Design review of the part built by this model. Coordinates are the model's own, in mm. A direction names the side the tool comes from. Round coordinates to 2 decimals unless told otherwise and drop trailing zeros. Loops run counter-clockwise (first coordinate to the right, second up) from the corner with the lowest first, then second, coordinate; pieces in that order, holes last. Notation, with made-up numbers: M 32.25,23.25 L 38.25,23.25 A29 ccw 38.25,51.25 Z; hole C 72,69.25 d1. An arc over 180 degrees is marked long. One line per item, written item: value. Start each with the question number.
Item 1: We need section C-C (x = 19). Write out the cut boundary in (y, z).
Item 2: Clearance check with a flat-ended pin moving along its axis: pin 1 (1.5 mm diameter, centred on x = -19.5, y = 23.5, fed in from +Z). State where the tip first meets the part, or that it passes through.
Item 3: For faces 1 (the flat face through (-18, 36.594, 31)), 2 (the flat face through (-68.472, -2, 28)), list the 3-axis set-ups (+Z, -Z, +X, -X, +Y, -Y) from which the entire face can be reached by the end or side of a thin tool; tool diameter is ignored.
Item 4: For line 1 along Y through (x, z) = (2.5, 17.5); line 2 along X through (y, z) = (-20, 40); line 3 along Z through (x, y) = (-32, -36), list the stretches that pass through material, from the lowest coordinate up.
Item 5: We need section A-A (z = 9.5). Write out the cut boundary in (x, y).
Item 6: Mouldability with a two-part tool opening along Y and no side actions: class faces 3 (the flat face through (-18, -46.271, 28)), 4 (the flat face through (-16, -41.152, 31)), 5 (the flat face through (-17, 41.641, 28)), 6 (the flat face through (-62.202, -3, 31)) as released by +Y, released by -Y, zero draft, split by the parting line, or undercut.
Item 7: We need section B-B (y = -36). Write out the cut boundary in (x, z), then the cut area to 3 significant figures.
from build123d import *

# Parameters (mm, degrees)
F0_W     = 90.4587376863
F0_H     = 77.7452811599
F1_DEPTH = 6.35
F0_W_2   = 5.1199775189
F2_DEPTH = 55.88


with BuildPart() as f1:
    # F0 (on Top) → F1 (new body)
    with BuildSketch(Plane.XY):
        with Locations((-16.9725483283, -2.2788867354)):
            Rectangle(F0_W, F0_H)
    extrude(amount=F1_DEPTH)

    # F0 (on Top) → F2 (join)
    with BuildSketch(Plane.XY):
        Polygon((-62.2019171715, 41.6413508356), (-62.2019171715, 36.5937538445), (28.2568205148, 36.5937538445), (33.3767980337, 36.5937538445), (33.3767980337, 41.6413508356), align=None)
        Polygon((-62.2019171715, -41.1515273154), (-62.2019171715, 36.5937538445), (-62.2019171715, 41.6413508356), (-68.4723928571, 41.6413508356), (-68.4723928571, -46.2711900473), (-62.2019171715, -46.2711900473), align=None)
        with Locations((30.8168092743, -2.2788867354)):
            Rectangle(F0_W_2, F0_H)
        Polygon((28.2568205148, -41.1515273154), (-62.2019171715, -41.1515273154), (-62.2019171715, -46.2711900473), (33.3767980337, -46.2711900473), (33.3767980337, -41.1515273154), align=None)
    extrude(amount=F2_DEPTH)


solid = f1.part
A:
1. outline: M -46.27,0 L 41.64,0 L 41.64,55.88 L 36.59,55.88 L 36.59,6.35 L -41.15,6.35 L -41.15,55.88 L -46.27,55.88 Z
2. pin 1: z = 6.35
3. face 1: +Z
3. face 2: +Z, -Z, -X, +Y, -Y
4. line 1: -46.27 to -41.15, 36.59 to 41.64
4. line 2: -68.47 to -62.2, 28.26 to 33.38
4. line 3: 0 to 6.35
5. outline: M -68.47,-46.27 L 33.38,-46.27 L 33.38,41.64 L -68.47,41.64 Z; hole M -62.2,-41.15 L 28.26,-41.15 L 28.26,36.59 L -62.2,36.59 Z
6. face 3: released by -Y
6. face 4: undercut
6. face 5: released by +Y
6. face 6: undercut
7. outline: M -68.47,0 L 33.38,0 L 33.38,55.88 L 28.26,55.88 L 28.26,6.35 L -62.2,6.35 L -62.2,55.88 L -68.47,55.88 Z
7. area: 1,210 mm2
